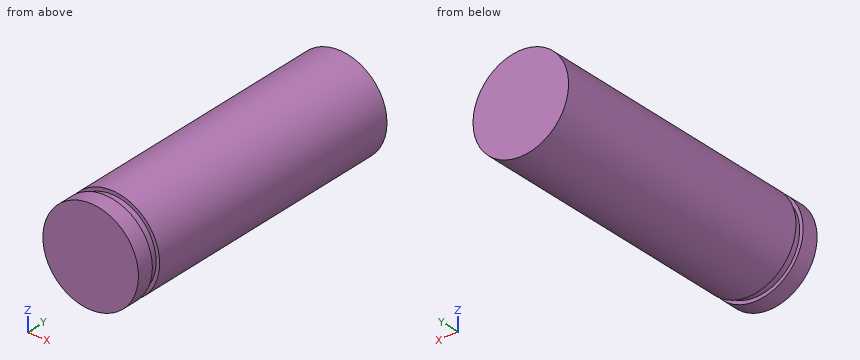
```python
from build123d import *

# Parameters (mm, degrees)
F0_R     = 3.9751
F1_DEPTH = 25.4
F3_R     = 7.385751
F3_R_2   = 3.683
F4_DEPTH = 0.7366


with BuildPart() as f1:
    # F0 (on Front) → F1 (new body)
    with BuildSketch(Plane.XZ):
        Circle(F0_R)
    extrude(amount=F1_DEPTH)

    # F3 (on offset) → F4 (cut)
    with BuildSketch(Plane.XZ.offset(23.241)):
        Circle(F3_R)
        Circle(F3_R_2, mode=Mode.SUBTRACT)
    extrude(amount=F4_DEPTH, mode=Mode.SUBTRACT)


solid = f1.part
```
Design review of the part built by this model. Coordinates are the model's own, in mm. Coordinates: 2 decimals unless noted, no trailing zeros. Write each loop counter-clockwise with the first axis right and the second up, starting at its lowest first coordinate (ties: lowest second). Pieces come first, ordered by that corner, then holes.
1) Add section C-C (y = -15.75). Write out the cut boundary in (x, z), plus the area to 3 significant figures.
2) Add section A-A (z = 2.25). Write out the cut boundary in (x, y), plus the area to 3 significant figures.
3) Insertion check: pin 1 (1 mm diameter, centred on y = -20.5, z = -3, fed in from -X); pin 2 (4 mm diameter, centred on x = 1.5, z = -0.5, fed in from +Y); pin 3 (3 mm diameter, centred on y = -3.5, z = 2.5, fed in from -X). Each pin has a flat end and moves straight along its axis. Give the tip position at first contact, or say it passes through.
4) To check wall thickness, follow L1, parallel to Z at x = -1.5, y = -11.25; L2, parallel to X at y = -13.75, z = 1. State the ranges of each line that lie inside material, in increasing order.
5) Add section B-B (x = -1.5). Write out the cut boundary in (y, z), plus the area to 3 significant figures.
Check result:
1. outline: circle Ø7.95 at (0, 0)
1. area: 49.6 mm2
2. outline: (-3.28, -25.4) - (3.28, -25.4) - (3.28, -23.98) - (2.92, -23.98) - (2.92, -23.24) - (3.28, -23.24) - (3.28, 0) - (-3.28, 0) - (-3.28, -23.24) - (-2.92, -23.24) - (-2.92, -23.98) - (-3.28, -23.98) - close
2. area: 166 mm2
3. pin 1: stops at x = -3.09
3. pin 2: stops at y = 0
3. pin 3: stops at x = -3.85
4. L1: z = -3.68 to 3.68
4. L2: x = -3.85 to 3.85
5. outline: (-25.4, -3.68) - (-23.98, -3.68) - (-23.98, -3.36) - (-23.24, -3.36) - (-23.24, -3.68) - (0, -3.68) - (0, 3.68) - (-23.24, 3.68) - (-23.24, 3.36) - (-23.98, 3.36) - (-23.98, 3.68) - (-25.4, 3.68) - close
5. area: 187 mm2
